Geometry: final body of the model. Coordinates: model frame, mm. Give positions to 0.01 mm unless a question says otherwise; leave off trailing zeros. Write each loop counter-clockwise with the first axis right and the second up, starting at its lowest first coordinate (ties: lowest second). Pieces come first, ordered by that corner, then holes.
from build123d import *
from build123d import SkipClean  # not in build123d's __all__

# Parameters (mm, degrees)
F1_DEPTH = 19.05
F2_DEPTH = 12.7
F3_DEPTH = 12.7


with BuildPart() as f1:
    # F0 (on Front) → F1 (new body)
    with BuildSketch(Plane.XZ):
        with BuildLine():
            ThreePointArc((61.5727165116, -19.0499999988), (61.5728220467, -19.0499999997), (61.5729275818, -19.05))
            ThreePointArc((61.5729275818, -19.05), (61.6368837688, -19.0498926403), (61.7008392349, -19.0495705623))
            ThreePointArc((61.7008392349, -19.0495705623), (80.6228005597, 0.0695667009), (61.5617064856, 19.0499966952))
            ThreePointArc((61.5617064856, 19.0499966952), (61.5090769294, 19.0498929943), (61.4564478606, 19.0496438936))
            ThreePointArc((61.4564478606, 19.0496438936), (42.4051790983, 0.0593448366), (61.3370395323, -19.0499973876))
            Line((61.3370395323, -19.0499973876), (61.5727165116, -19.0499999988))
        make_face()
        with BuildLine():
            ThreePointArc((61.5729275818, -12.7), (52.5926714608, 8.9802561211), (74.2729275818, 0))
            ThreePointArc((74.2729275818, 0), (70.5531837029, -8.9802561211), (61.5729275818, -12.7))
        make_face(mode=Mode.SUBTRACT)
        with BuildLine():
            ThreePointArc((61.3370395323, -19.0499973876), (61.4548780179, -19.0503631562), (61.5727165116, -19.0499999988))
            Line((61.5727165116, -19.0499999988), (61.3370395323, -19.0499973876))
        make_face()
        with BuildLine():
            ThreePointArc((61.5617064856, 19.0499966952), (80.6228005597, 0.0695667009), (61.7008392349, -19.0495705623))
            Line((61.7008392349, -19.0495705623), (105.7561740171, -18.7537533585))
            ThreePointArc((105.7561740171, -18.7537533585), (124.6268697008, 0.4243875569), (105.5006242064, 19.3476794968))
            Line((105.5006242064, 19.3476794968), (61.5617064856, 19.0499966952))
        make_face()
        with BuildLine():
            Line((17.5163885853, -19.0495118633), (61.3370395323, -19.0499973876))
            ThreePointArc((61.3370395323, -19.0499973876), (42.4051790983, 0.0593448366), (61.4564478606, 19.0496438936))
            Line((61.4564478606, 19.0496438936), (17.516521874, 19.0527779802))
            ThreePointArc((17.516521874, 19.0527779802), (-1.4824426783, 0.0016995201), (17.5163885853, -19.0495118633))
        make_face()
        with BuildLine():
            ThreePointArc((61.5729275818, -12.7), (70.5531837029, -8.9802561211), (74.2729275818, 0))
            ThreePointArc((74.2729275818, 0), (52.5926714608, 8.9802561211), (61.5729275818, -12.7))
        make_face()
        with BuildLine():
            ThreePointArc((67.9229275818, 0), (66.0630556424, -4.4901280605), (61.5729275818, -6.35))
            ThreePointArc((61.5729275818, -6.35), (57.0827995213, 4.4901280605), (67.9229275818, 0))
        make_face(mode=Mode.SUBTRACT)
    extrude(amount=F1_DEPTH)

    # F0 (on Front) → F2 (cut)
    with BuildSketch(Plane.XZ):
        with BuildLine():
            ThreePointArc((61.5729275818, -12.7), (70.5531837029, -8.9802561211), (74.2729275818, 0))
            ThreePointArc((74.2729275818, 0), (52.5926714608, 8.9802561211), (61.5729275818, -12.7))
        make_face()
        with BuildLine():
            ThreePointArc((67.9229275818, 0), (66.0630556424, -4.4901280605), (61.5729275818, -6.35))
            ThreePointArc((61.5729275818, -6.35), (57.0827995213, 4.4901280605), (67.9229275818, 0))
        make_face(mode=Mode.SUBTRACT)
        with BuildLine():
            Line((17.5163885853, -19.0495118633), (61.3370395323, -19.0499973876))
            ThreePointArc((61.3370395323, -19.0499973876), (42.4051790983, 0.0593448366), (61.4564478606, 19.0496438936))
            Line((61.4564478606, 19.0496438936), (17.516521874, 19.0527779802))
            ThreePointArc((17.516521874, 19.0527779802), (-1.4824426783, 0.0016995201), (17.5163885853, -19.0495118633))
        make_face()
    extrude(amount=F2_DEPTH, mode=Mode.SUBTRACT)

    # F0 (on Front) → F3 (cut)
    with BuildSketch(Plane.XZ):
        with BuildLine():
            ThreePointArc((61.5617064856, 19.0499966952), (80.6228005597, 0.0695667009), (61.7008392349, -19.0495705623))
            Line((61.7008392349, -19.0495705623), (105.7561740171, -18.7537533585))
            ThreePointArc((105.7561740171, -18.7537533585), (124.6268697008, 0.4243875569), (105.5006242064, 19.3476794968))
            Line((105.5006242064, 19.3476794968), (61.5617064856, 19.0499966952))
        make_face()
    with SkipClean():  # cleaning this boolean's faces spoils the solid; the shape is the same uncleaned
        extrude(amount=F3_DEPTH, mode=Mode.SUBTRACT)


solid = f1.part
Q1. Ray query, line 1 along Y through (x, z) = (31, -4); line 2 along X through (y, z) = (-6, 0); line 3 along X through (y, z) = (-10, 5). Return the intervals inside material, ascending.
Filled sheet:
line 1: y = -19.05 to -12.7
line 2: x = 42.41 to 48.87, 74.27 to 80.62
line 3: x = 43.07 to 49.9, 73.25 to 79.96
Q2. Section B-B on z = -3. Output: boundary loops of the cut face in (x, y).
Filled sheet:
outline: (-1.24, -19.05) - (55.98, -19.05) - (55.98, -12.7) - (49.23, -12.7) - (49.23, 0) - (42.64, 0) - (42.64, -12.7) - (-1.24, -12.7) - close; (67.17, -19.05) - (124.34, -19.05) - (124.34, -12.7) - (80.39, -12.7) - (80.39, 0) - (73.91, 0) - (73.91, -12.7) - (67.17, -12.7) - close
Q3. Pin query (flat end, axial travel): P1, Ø8, axis at y = -8.5, z = 3.5, coming from the +X side; P2, Ø19, axis at x = 105.5, z = -8.5, coming from the +Y side; P3, Ø5, axis at y = -7.5, z = 8, coming from the +X side; P4, Ø7.5, axis at x = 61.57, z = 0, coming from the +Y side. Return the tip coordinate at first contact, or that it passes through.
Filled sheet:
P1: stops at x = 80.62
P2: stops at y = -12.7
P3: stops at x = 79.81
P4: passes through
Q4. Section D-D on z = 16. Output: boundary loops of the cut face in (x, y).
Filled sheet:
outline: (7.22, -19.05) - (116.36, -19.05) - (116.36, -12.7) - (71.91, -12.7) - (71.91, 0) - (51.12, 0) - (51.12, -12.7) - (7.22, -12.7) - close
Q5. Pull-direction query (X, two-part tool) for faces 1 (the cylindrical face through (-1.478, -15.831, 0.42)), 2 (the flat face through (100, -12.7, 0)), 3 (the flat face through (59, -12.7, 6)); classes: released by +X, released by -X, zero draft, split by the parting line, or undercut.
Filled sheet:
face 1: released by -X
face 2: zero draft
face 3: undercut
